Read the model definition and answer for the solid it produces. Units are mm, in the model's axes. A direction names the side the tool comes from. Round coordinates to 2 decimals unless told otherwise and drop trailing zeros. Write each loop counter-clockwise with the first axis right and the second up, starting at its lowest first coordinate (ties: lowest second). Pieces come first, ordered by that corner, then holes. Notation, with made-up numbers: (44.25, 39.5) - (96.25, 39.5) arc R22 ccw to (96.25, 58.5) - close; hole circle Ø8 at (67.25, 29). An arc over 180 degrees is marked (long way). Answer as CSV lines item,"result". Start each with the question number.
1) Consider line 1 along Y through (x, z) = (0, -6.5); line 2 along X through (y, z) = (0, 4.75); line 3 along Z through (x, y) = (-12.5, -4.5). Determine where each line is inside the solid, lowest interval first.
2) Each of these flat-tipped pins is pushed along its axis until it touches: pin 1 (2 mm diameter, centred on x = 7, z = 5.5, fed in from -Y); pin 2 (4 mm diameter, centred on y = -3.5, z = 0, fed in from +X); pin 3 (4 mm diameter, centred on x = -8.5, z = 3.5, fed in from -Y); pin 4 (2.5 mm diameter, centred on x = 0, y = 16.5, fed in from -Z). Where does it stop, or does it pass through?
3) Find section B-B on y = 0. Determine the outline of the cut face in (x, z).
4) For a pull along Y with two mould halves and no side action, classify faces 1 (the cylindrical face through (11.446, 3.604, 6.451)), 2 (the flat face through (9, -9, 3)), 3 (the cylindrical face through (0.9, -18.23, -3.9)) as +Y half, -Y half, draft (parallel to the pull), parting line (faces both ways), or undercut.
5) Find section A-A on x = 0. Determine the outline of the cut face in (y, z), then the cut area to 3 significant figures.
6) Find section D-D on x = 8. Determine the outline of the cut face in (y, z), then the cut area to 3 significant figures.
7) Find section C-C on z = 6.5. Determine the outline of the cut face in (x, y).
8) Which of the six approach directions +Z, -Z, +X, -X, +Y, -Y give full straight-line access (tool end or side, diameter ignored) to faces 4 (the cylindrical face through (5, 7.84, -5.42)), 5 (the cylindrical face through (20.03, 6.31, -3.9))?
from build123d import *

# Parameters (mm, degrees)
F0_R     = 21
F0_R_2   = 12
F0_R_3   = 4.1
F1_DEPTH = 3
F2_DEPTH = 10
F3_R     = 21
F3_R_2   = 9.3
F4_DEPTH = 11
F5_R     = 1.95
F6_DEPTH = 14
F7_R     = 1
F8_DEPTH = 12.5


with BuildPart() as f1:
    # F0 (on Top) → F1 (new body)
    with BuildSketch(Plane.XY):
        Circle(F0_R)
        Circle(F0_R_2, mode=Mode.SUBTRACT)
        Circle(F0_R_2)
        Circle(F0_R_3, mode=Mode.SUBTRACT)
    extrude(amount=F1_DEPTH)

    # F0 (on Top) → F2 (join)
    with BuildSketch(Plane.XY):
        Circle(F0_R_2)
        Circle(F0_R_3, mode=Mode.SUBTRACT)
    extrude(amount=F2_DEPTH)

    # F3 (on Top) → F4 (join)
    with BuildSketch(Plane.XY):
        Circle(F3_R)
        Circle(F3_R_2, mode=Mode.SUBTRACT)
    extrude(amount=-F4_DEPTH)

    # F5 (on face) → F6 (cut, through all)
    with BuildSketch(Plane.XY.offset(3)):
        with Locations((0, 16.5)):
            Circle(F5_R)
        with Locations((0, -16.5)):
            Circle(F5_R)
    extrude(amount=-F6_DEPTH, mode=Mode.SUBTRACT)

    # F7 (on Right) → F8 (cut, symmetric)
    with BuildSketch(Plane.YZ):
        with Locations((0, 6.5)):
            Circle(F7_R)
    extrude(amount=F8_DEPTH, both=True, mode=Mode.SUBTRACT)


solid = f1.part
Check values:
1,line 1,"y = -21 to -18.45, -14.55 to -9.3, 9.3 to 14.55, 18.45 to 21"
1,line 2,"x = -12 to -4.1, 4.1 to 12"
1,line 3,"z = -11 to 3"
2,pin 1,"stops at y = -10.39"
2,pin 2,"stops at x = 20.95"
2,pin 3,"stops at y = -19.95"
2,pin 4,"passes through"
3,outline,"(-21, -11) - (-9.3, -11) - (-9.3, 0) - (-4.1, 0) - (-4.1, 5.5) - (-12, 5.5) - (-12, 3) - (-21, 3) - close; (-12, 7.5) - (-4.1, 7.5) - (-4.1, 10) - (-12, 10) - close; (4.1, 0) - (9.3, 0) - (9.3, -11) - (21, -11) - (21, 3) - (12, 3) - (12, 5.5) - (4.1, 5.5) - close; (4.1, 7.5) - (12, 7.5) - (12, 10) - (4.1, 10) - close"
4,face 1,"parting line"
4,face 2,"draft"
4,face 3,"undercut"
5,outline,"(-21, -11) - (-18.45, -11) - (-18.45, 3) - (-21, 3) - close; (-14.55, -11) - (-9.3, -11) - (-9.3, 0) - (-4.1, 0) - (-4.1, 10) - (-12, 10) - (-12, 3) - (-14.55, 3) - close; (4.1, 0) - (9.3, 0) - (9.3, -11) - (14.55, -11) - (14.55, 3) - (12, 3) - (12, 10) - (4.1, 10) - close; (18.45, -11) - (21, -11) - (21, 3) - (18.45, 3) - close"
5,area,"360 mm^2"
6,outline,"(-19.42, -11) - (-4.74, -11) - (-4.74, 0) - (4.74, 0) - (4.74, -11) - (19.42, -11) - (19.42, 3) - (8.94, 3) - (8.94, 10) - (-8.94, 10) - (-8.94, 3) - (-19.42, 3) - close; hole circle Ø2 at (0, 6.5)"
6,area,"561 mm^2"
7,outline,"(-11.96, -1) arc R12 ccw to (11.96, -1) - (3.98, -1) arc R4.1 cw to (-3.98, -1) - close; (-11.96, 1) - (-3.98, 1) arc R4.1 cw to (3.98, 1) - (11.96, 1) arc R12 ccw to start"
8,face 4,"-Z"
8,face 5,"+Z, -Z"
